Verification items for the finished model (mm, model axes). Face numbers are marked on the shaded views. A direction names the side the tool comes from. Coordinates: 2 decimals unless noted, no trailing zeros. Order: outer loops, then holes, each group sorted by start corner. A loop starts at its lowest first (then second) coordinate and runs counter-clockwise, first axis right, second up. Notation, with made-up numbers: M 14,11 L 70,11 A10 ccw 70,19 Z; hole C 19.25,-5 d8. An arc over 180 degrees is marked long. Answer as a JSON object with one key per item and string values. Group by question number.
(1) Cross-section at C-C (z = -10.5). Enter the section's corners in (x, y), plus the area to 3 significant figures.
(2) Cross-section at B-B (x = -12). Enter the section's corners in (y, z).
(3) Access from +Z, -Z, +X, -X, +Y, -Y to the whole of each face (thin tool, end or side, straight path). Record for the marked faces 1, 2 and 3.
(4) Material ranges on line 1 (Y direction, x = -12, z = -14.65); line 2 (Y direction, x = 14, z = -15); line 3 (X direction, y = 5, z = -3), recorded low to high.
(5) Gauge pin test, flat ends, axial feed: pin 1 Ø4 at (y, z) = (8.5, -12) entering from +X; pin 2 Ø1.3 at (x, z) = (11, -5) entering from -Y; pin 3 Ø6 at (x, y) = (-13.5, 0.5) entering from +Z; pin 4 Ø0.7 at (y, z) = (1.5, 0.5) entering from +X. Record the tip position at first contact, or that the pin passes through.
(6) Cross-section at D-D (x = 11). Enter the section's corners in (y, z).
(7) Mould release check, pull along Z, two halves, no side actions. Record for the marked faces 4, 5, 6 and 7: released by +Z, released by -Z, zero draft, split by the parting line, or undercut.
(8) Cross-section at A-A (z = 8). Enter the section's corners in (x, y) (3 decimals).
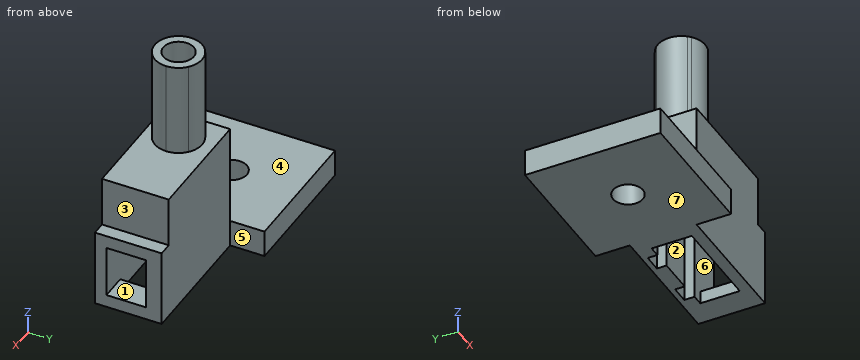
from build123d import *

# Parameters (mm, degrees)
SKETCH1_W           = 17.4
SKETCH1_H           = 9.850463562
BOSS_EXTRUDE1_DEPTH = 2
BOSS_EXTRUDE2_START = 1.9
SKETCH1_4_R         = 2.25
BOSS_EXTRUDE2_DEPTH = 14
SKETCH2_W           = 17.4
SKETCH2_H           = 9.850463562
BOSS_EXTRUDE3_DEPTH = 17
SKETCH4_W           = 7.7
SKETCH4_H           = 5.83
CUT_EXTRUDE1_DEPTH  = 1.9
SKETCH5_W           = 20
SKETCH5_H           = 20
SKETCH5_R           = 2.2
BOSS_EXTRUDE4_DEPTH = 4
CHAMFER1_SIZE       = 0.5
SKETCH6_W           = 11.54
SKETCH6_H           = 9.850463562
SKETCH6_W_2         = 7.7
SKETCH6_H_2         = 5.83
BOSS_EXTRUDE5_DEPTH = 2


with BuildPart() as part:
    # Sketch1 → Boss-Extrude1 (new body)
    with BuildSketch(Plane.XY):
        with Locations((6.7, 2.924768219)):
            Rectangle(SKETCH1_W, SKETCH1_H)
        with BuildLine():
            Line((0, 0.396129135), (0, 4.933870865))
            ThreePointArc((0, 4.933870865), (0.190126266, 5.139873734), (0.396129135, 5.33))
            Line((0.396129135, 5.33), (4.933870865, 5.33))
            ThreePointArc((4.933870865, 5.33), (6.165, 2.665), (4.933870865, 0))
            Line((4.933870865, 0), (0.396129135, 0))
            ThreePointArc((0.396129135, 0), (0.190126266, 0.190126266), (0, 0.396129135))
        make_face(mode=Mode.SUBTRACT)
    extrude(amount=BOSS_EXTRUDE1_DEPTH)

    # Sketch1<4> → Boss-Extrude2 (add)
    # profile 1 of 4: a face of its own
    with BuildSketch(Plane.XY.offset(BOSS_EXTRUDE2_START)):
        with BuildLine():
            ThreePointArc((0.396129135, 5.33), (0.190126266, 5.139873734), (0, 4.933870865))
            Line((0, 4.933870865), (0, 0.396129135))
            ThreePointArc((0, 0.396129135), (0.190126266, 0.190126266), (0.396129135, 0))
            Line((0.396129135, 0), (4.933870865, 0))
            ThreePointArc((4.933870865, 0), (5.842345435, 1.197186665), (6.165, 2.665))
            ThreePointArc((6.165, 2.665), (5.842345435, 4.132813335), (4.933870865, 5.33))
            Line((4.933870865, 5.33), (0.396129135, 5.33))
        make_face()
        with Locations((2.665, 2.665)):
            Circle(SKETCH1_4_R, mode=Mode.SUBTRACT)
    # profile 2 of 4: a face of its own
    with BuildSketch(Plane.XY.offset(BOSS_EXTRUDE2_START)):
        with BuildLine():
            Line((0, 0.396129135), (0, 4.933870865))
            ThreePointArc((0, 4.933870865), (-0.835, 2.665), (0, 0.396129135))
        make_face()
    # profile 3 of 4: a face of its own
    with BuildSketch(Plane.XY.offset(BOSS_EXTRUDE2_START)):
        with BuildLine():
            ThreePointArc((4.933870865, 5.33), (2.665, 6.165), (0.396129135, 5.33))
            Line((0.396129135, 5.33), (4.933870865, 5.33))
        make_face()
    # profile 4 of 4: a face of its own
    with BuildSketch(Plane.XY.offset(BOSS_EXTRUDE2_START)):
        with BuildLine():
            Line((4.933870865, 0), (0.396129135, 0))
            ThreePointArc((0.396129135, 0), (2.665, -0.835), (4.933870865, 0))
        make_face()
    extrude(amount=BOSS_EXTRUDE2_DEPTH)

    # Sketch2 → Boss-Extrude3 (add)
    with BuildSketch(Plane(origin=(0, 0, 0), x_dir=(-1, 0, 0), z_dir=(0, 0, -1))):
        with Locations((-6.7, 2.924768219)):
            Rectangle(SKETCH2_W, SKETCH2_H)
        Polygon((-13.5, 5.53), (-11.88, 5.53), (-11.88, 7.05), (-9.28, 7.05), (-9.28, 5.63), (-4.12, 5.63), (-4.12, 7.05), (-1.52, 7.05), (-1.52, 5.63), (0.1, 5.63), (0.1, -0.3), (-13.5, -0.3), align=None, mode=Mode.SUBTRACT)
    extrude(amount=BOSS_EXTRUDE3_DEPTH)

    # Sketch4 → Cut-Extrude1 (cut)
    with BuildSketch(Plane.ZY.offset(-13.5)):
        with Locations((-11.23, 2.615)):
            Rectangle(SKETCH4_W, SKETCH4_H)
    extrude(amount=-CUT_EXTRUDE1_DEPTH, mode=Mode.SUBTRACT)

    # Sketch5 → Boss-Extrude4 (add)
    with BuildSketch(Plane(origin=(0, 0, -17), x_dir=(-1, 0, 0), z_dir=(0, 0, -1))):
        with Locations((12, 2.924768219)):
            Rectangle(SKETCH5_W, SKETCH5_H)
        with Locations((12, 2.924768219)):
            Circle(SKETCH5_R, mode=Mode.SUBTRACT)
    extrude(amount=-BOSS_EXTRUDE4_DEPTH)

    # Chamfer1
    # the kernel refuses this chamfer: 0.5 mm, written as the material it adds along each edge
    with BuildSketch(Plane(origin=(0, -0.889712359, 1.9), x_dir=(-0.027495876610586365, 0, -0.9996219169112968), z_dir=(0, 1, 0))) as chamfer1_piece_1_section:
        Polygon((CHAMFER1_SIZE * 0.999621916911, -CHAMFER1_SIZE * 0.0274958766106), (-CHAMFER1_SIZE * 0.0274958766106, -CHAMFER1_SIZE * 0.999621916911), (0, 0), align=None)
    chamfer1_piece_1 = extrude(amount=7.109424717, mode=Mode.PRIVATE)
    chamfer1_piece_1 = chamfer1_piece_1 - Plane(origin=(2.665, 2.665, 1.727474794), x_dir=(1, 0, 0), z_dir=(0, 0, -1)) * Cylinder(2.25, 17, mode=Mode.PRIVATE)
    add(chamfer1_piece_1)
    with BuildSketch(Plane(origin=(-0.889712359, 5.33, 1.9), x_dir=(0, 0.027495876610585623, -0.9996219169112968), z_dir=(1, 0, 0))) as chamfer1_piece_2_section:
        Polygon((CHAMFER1_SIZE * 0.999621916911, -CHAMFER1_SIZE * 0.0274958766106), (-CHAMFER1_SIZE * 0.0274958766106, -CHAMFER1_SIZE * 0.999621916911), (0, 0), align=None)
    chamfer1_piece_2 = extrude(amount=7.109424717, mode=Mode.PRIVATE)
    chamfer1_piece_2 = chamfer1_piece_2 - Plane(origin=(2.665, 2.665, 1.727474794), x_dir=(1, 0, 0), z_dir=(0, 0, -1)) * Cylinder(2.25, 17, mode=Mode.PRIVATE)
    add(chamfer1_piece_2)
    with BuildSketch(Plane(origin=(6.219712359, 0, 1.9), x_dir=(0, -0.027495876610586365, -0.9996219169112968), z_dir=(-1, 0, 0))) as chamfer1_piece_3_section:
        Polygon((CHAMFER1_SIZE * 0.999621916911, -CHAMFER1_SIZE * 0.0274958766106), (-CHAMFER1_SIZE * 0.0274958766106, -CHAMFER1_SIZE * 0.999621916911), (0, 0), align=None)
    chamfer1_piece_3 = extrude(amount=7.109424717, mode=Mode.PRIVATE)
    chamfer1_piece_3 = chamfer1_piece_3 - Plane(origin=(2.665, 2.665, 1.727474794), x_dir=(1, 0, 0), z_dir=(0, 0, -1)) * Cylinder(2.25, 17, mode=Mode.PRIVATE)
    add(chamfer1_piece_3)
    with BuildSketch(Plane(origin=(2.665, 2.665, 1.9), x_dir=(-0.9434537391287974, -0.3315042113215022, 0), z_dir=(-0.3315042113215022, 0.9434537391287974, 0))) as chamfer1_piece_4:
        Polygon((3.5, -CHAMFER1_SIZE), (3.5 - CHAMFER1_SIZE, 0), (3.5, 0), align=None)
    revolve(axis=Axis((2.665, 2.665, 1.9), (0, 0, 1)), revolution_arc=51.27979911)
    with BuildSketch(Plane(origin=(2.665, 2.665, 1.9), x_dir=(0.33133655383280003, -0.943512632715749, 0), z_dir=(-0.943512632715749, -0.33133655383280003, 0))) as chamfer1_piece_5:
        Polygon((3.5, -CHAMFER1_SIZE), (3.5 - CHAMFER1_SIZE, 0), (3.5, 0), align=None)
    revolve(axis=Axis((2.665, 2.665, 1.9), (0, 0, 1)), revolution_arc=141.300162094)
    with BuildSketch(Plane(origin=(2.665, 2.665, 1.9), x_dir=(-0.33150421132149205, 0.9434537391288009, 0), z_dir=(0.9434537391288009, 0.33150421132149205, 0))) as chamfer1_piece_6:
        Polygon((3.5, -CHAMFER1_SIZE), (3.5 - CHAMFER1_SIZE, 0), (3.5, 0), align=None)
    revolve(axis=Axis((2.665, 2.665, 1.9), (0, 0, 1)), revolution_arc=51.27979911)

    # Sketch6 → Boss-Extrude5 (add)
    with BuildSketch(Plane(origin=(15.4, 0, 0), x_dir=(0, 0, -1), z_dir=(1, 0, 0))):
        with Locations((11.23, 2.924768219)):
            Rectangle(SKETCH6_W, SKETCH6_H)
        with Locations((11.23, 2.615)):
            Rectangle(SKETCH6_W_2, SKETCH6_H_2, mode=Mode.SUBTRACT)
    extrude(amount=BOSS_EXTRUDE5_DEPTH)


solid = part.part
Taken from the geometry:
{
 "1": {"outline": "M -2,-2 L 17.4,-2 L 17.4,-0.3 L -0.1,-0.3 L -0.1,5.63 L 1.52,5.63 L 1.52,7.05 L 4.12,7.05 L 4.12,5.63 L 9.28,5.63 L 9.28,7.05 L 11.88,7.05 L 11.88,5.53 L 17.4,5.53 L 17.4,7.85 L -2,7.85 Z", "area": "80.5 mm²"},
 "2": {"outline": "M -7.08,-17 L 0.72,-17 L 0.72,-13 L -7.08,-13 Z; M 5.12,-17 L 12.92,-17 L 12.92,-13 L 5.12,-13 Z"},
 "3": {"face 1": "+X", "face 2": "-Z", "face 3": "+Z, +X, +Y, -Y"},
 "4": {"line 1": "y = -7.08 to 0.72, 5.12 to 12.92", "line 2": "y = -2 to -0.3, 5.53 to 7.85", "line 3": "x = -2 to -0.1, 13.5 to 15.4"},
 "5": {"pin 1": "stops at x = 17.4", "pin 2": "stops at y = -2", "pin 3": "stops at z = -13", "pin 4": "stops at x = 15.4"},
 "6": {"outline": "M -2,-17 L -0.3,-17 L -0.3,0 L 7.05,0 L 7.05,-17 L 7.85,-17 L 7.85,2 L -2,2 Z"},
 "7": {"face 4": "released by +Z", "face 5": "zero draft", "face 6": "undercut", "face 7": "released by -Z"},
 "8": {"outline": "C 2.665,2.665 d7; hole C 2.665,2.665 d4.5"}
}
